Here's how the part is built. I have some questions about the finished solid (model axes, mm). Face numbers are marked on the shaded views. A direction names the side the tool comes from. Give positions to 0.01 mm unless a question says otherwise; leave off trailing zeros. Loops run counter-clockwise (first coordinate to the right, second up) from the corner with the lowest first, then second, coordinate; pieces in that order, holes last. Notation, with made-up numbers: (3.5, 3) - (23.5, 3) arc R9 cw to (23.5, 14) - close; hole circle Ø4 at (76.25, 8.25). An arc over 180 degrees is marked (long way). Return JSON: item names as keys, results as strings. Group by question number.
(1) I need wall thicknesses on probe 1 along X at (y, z) = (-5, -3.3); probe 2 along X at (y, z) = (-9.75, -1.8); probe 3 along Y at (x, z) = (10, -1.2). Which ranges of each line are inside material? Lowest first, please. Write a range as [from, to].
(2) If we mould it in two halves opening along X, with no side actions, what happens to the marked faces 1, 2, 3 and 4? For each: released by +X, released by -X, zero draft, split by the parting line, or undercut.
(3) If we section it at B-B (x = 6): Please give me the cut outline in (y, z).
(4) If we section it at A-A (z = -2.4): State how many separate pieces and enclosed holes the cut face has, then the cut area to 3 significant figures.
(5) For P1, Ø4, axis at x = 12, y = -19.5, coming from the -Z side, with a flat end and sliding along its axis, tell me the tip position at first contact or that it passes through.
(6) If we section it at C-C (y = -3.25): Please give me the cut outline in (x, z).
(7) On a 3-axis mill with a long thin cutter (end or side, diameter ignored), from which of +Z, -Z, +X, -X, +Y, -Y can I reach the whole of each face in a straight line? I mean the marked faces 5 and 6. Say none if no direction works.
(8) If we section it at D-D (y = -16): Please give me the cut outline in (x, z), then the cut area to 3 significant figures.
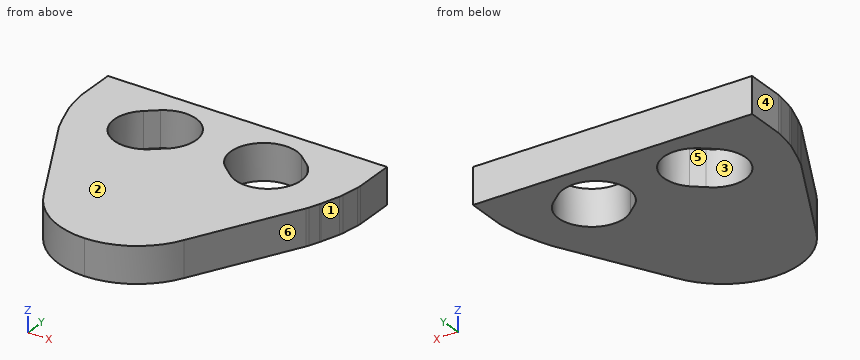
```python
from build123d import *

# Parameters (mm, degrees)
F1_DEPTH = 4


with BuildPart() as f1:
    # F0 (on Top) → F1 (new body)
    with BuildSketch(Plane.XY):
        with BuildLine():
            Line((0, -23.741776), (0, 0))
            Line((0, 0), (-12.5, 0))
            Line((-12.5, 0), (-15.5, 0))
            Line((-15.5, 0), (-15.5, -4.3325))
            Line((-15.5, -4.3325), (-15.457999, -4.832742))
            Line((-15.457999, -4.832742), (-15.141206, -6.705982))
            Line((-15.141206, -6.705982), (-15.029257, -7.154422))
            Line((-15.029257, -7.154422), (-14.352191, -9.185621))
            Line((-14.352191, -9.185621), (-14.295931, -9.340147))
            Line((-14.295931, -9.340147), (-13.870512, -10.415947))
            Line((-13.870512, -10.415947), (-13.734117, -10.712556))
            Line((-13.734117, -10.712556), (-7.782776, -21.993459))
            ThreePointArc((-7.782776, -21.993459), (-4.579278, -25.516799), (0, -26.823145))
            Line((0, -26.823145), (0, -23.741776))
        make_face()
        with BuildLine():
            Line((-9.056534, -3.694688), (-7.853357, -2.704581))
            ThreePointArc((-7.853357, -2.704581), (-2.840883, -3.156518), (-3.007137, -8.186578))
            Line((-3.007137, -8.186578), (-4.200585, -9.17746))
            ThreePointArc((-4.200585, -9.17746), (-9.471274, -8.953792), (-9.056534, -3.694688))
        make_face(mode=Mode.SUBTRACT)
    extrude(amount=-F1_DEPTH)

    # F2: F1 across plane


with BuildPart() as f1_1:
    add(f1.part)
    add(f1.part.mirror(Plane.YZ))


solid = f1_1.part
```
Values:
{
 "1": {"probe 1": "[-15.43, -10.06], [-1.97, 1.97], [10.06, 15.43]", "probe 2": "[-14.13, -8.47], [-4.99, 4.99], [8.47, 14.13]", "probe 3": "[-17.79, -8.17], [-4.87, 0]"},
 "2": {"face 1": "released by +X", "face 2": "zero draft", "face 3": "undercut", "face 4": "released by -X"},
 "3": {"outline": "(-24.42, -4) - (-10.12, -4) - (-10.12, 0) - (-24.42, 0) - close; (-1.94, -4) - (0, -4) - (0, 0) - (-1.94, 0) - close"},
 "4": {"separate pieces": "1", "enclosed holes": "2", "area": "514 mm2"},
 "5": {"P1": "through"},
 "6": {"outline": "(-15.5, -4) - (-8.52, -4) - (-8.52, 0) - (-15.5, 0) - close; (-2.76, -4) - (2.76, -4) - (2.76, 0) - (-2.76, 0) - close; (8.52, -4) - (15.5, -4) - (15.5, 0) - (8.52, 0) - close"},
 "7": {"face 5": "+Z, -Z", "face 6": "+Z, -Z, +X, -Y"},
 "8": {"outline": "(-10.94, -4) - (10.94, -4) - (10.94, 0) - (-10.94, 0) - close", "area": "87.6 mm2"}
}
